The model under review builds one solid part; all positions refer to its coordinate system, in mm. Coordinates: 2 decimals unless noted, no trailing zeros. Loops run counter-clockwise (first coordinate to the right, second up) from the corner with the lowest first, then second, coordinate; pieces in that order, holes last. Notation, with made-up numbers: M 69,29.5 L 76,29.5 A25 ccw 76,52.5 Z; hole C 4,-10 d4. An arc over 180 degrees is marked long. Return JSON: item names as keys, results as strings.
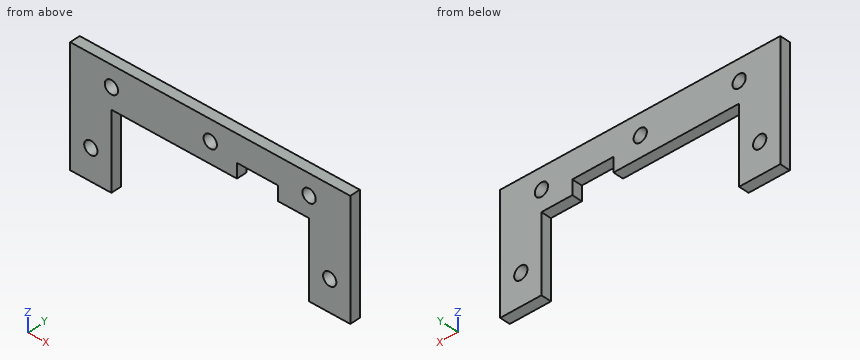
```python
from build123d import *

# Parameters (mm, degrees)
BOSS_EXTRUDE1_DEPTH = 5
SKETCH3_W           = 20
SKETCH3_H           = 7
CUT_EXTRUDE1_DEPTH  = 130.344501236
SKETCH4_R           = 3.225
CUT_EXTRUDE2_DEPTH  = 130.344501236


with BuildPart() as part:
    # Sketch2 → Boss-Extrude1 (new body)
    with BuildSketch(Plane(origin=(0, 0, 0), x_dir=(1, 0, 0), z_dir=(0, 1, 0))):
        Polygon((0, 0), (-20, 0), (-20, -57), (116, -57), (116, 0), (96, 0), (96, -37), (0, -37), align=None)
    extrude(amount=BOSS_EXTRUDE1_DEPTH)

    # Sketch3 → Cut-Extrude1 (cut, through all)
    with BuildSketch(Plane(origin=(0, 5, 0), x_dir=(1, 0, 0), z_dir=(0, 1, 0))):
        with Locations((71, -40.5)):
            Rectangle(SKETCH3_W, SKETCH3_H)
    extrude(amount=-CUT_EXTRUDE1_DEPTH, mode=Mode.SUBTRACT)

    # Sketch4 → Cut-Extrude2 (cut, through all)
    with BuildSketch(Plane(origin=(0, 5, 0), x_dir=(1, 0, 0), z_dir=(0, 1, 0))):
        with Locations(Location((-10, -15, 0), (0, 0, 270))):
            Circle(SKETCH4_R)
        with Locations(Location((0, -47, 0), (0, 0, 270))):
            Circle(SKETCH4_R)
        with Locations(Location((48, -47, 0), (0, 0, 270))):
            Circle(SKETCH4_R)
        with Locations(Location((96, -47, 0), (0, 0, 270))):
            Circle(SKETCH4_R)
        with Locations(Location((106, -15, 0), (0, 0, 270))):
            Circle(SKETCH4_R)
    extrude(amount=-CUT_EXTRUDE2_DEPTH, mode=Mode.SUBTRACT)


solid = part.part
```
1. To check wall thickness, follow line 1 (X direction, y = 1.95, z = 47) (3 decimals); line 2 (X direction, y = 1.95, z = 15) (3 decimals); line 3 (X direction, y = 1, z = 32). State the ranges of each line that lie inside material, in increasing order.
Check values:
{"line 1": "-20 to -3.225, 3.225 to 44.775, 51.225 to 92.775, 99.225 to 116", "line 2": "-20 to -13.225, -6.775 to 0, 96 to 102.775, 109.225 to 116", "line 3": "-20 to 0, 96 to 116"}
2. Add section B-B on z = 15. Give the boundary of the cut face in (x, y) (3 decimals).
Check values:
{"outline": "M -20,0 L -13.225,0 L -13.225,5 L -20,5 Z; M -6.775,0 L 0,0 L 0,5 L -6.775,5 Z; M 96,0 L 102.775,0 L 102.775,5 L 96,5 Z; M 109.225,0 L 116,0 L 116,5 L 109.225,5 Z"}
3. Add section D-D on y = 2.3. Give the boundary of the cut face in (x, z) (3 decimals).
Check values:
{"outline": "M -20,0 L 0,0 L 0,37 L 61,37 L 61,44 L 81,44 L 81,37 L 96,37 L 96,0 L 116,0 L 116,57 L -20,57 Z; hole C -10,15 d6.45; hole C 0,47 d6.45; hole C 48,47 d6.45; hole C 96,47 d6.45; hole C 106,15 d6.45"}
4. Add section A-A on x = 48. Give the boundary of the cut face in (y, z) (3 decimals).
Check values:
{"outline": "M 0,37 L 5,37 L 5,43.775 L 0,43.775 Z; M 0,50.225 L 5,50.225 L 5,57 L 0,57 Z"}
5. Add section C-C on z = 41.5. Give the boundary of the cut face in (x, y).
Check values:
{"outline": "M -20,0 L 61,0 L 61,5 L -20,5 Z; M 81,0 L 116,0 L 116,5 L 81,5 Z"}
